```python
from build123d import *

# Parameters (mm, degrees)
SKETCH_1_R           = 11
EXTRUDE_1_DEPTH      = 50
SKETCH_2_R           = 7.5
CUT_EXTRUDE_1_DEPTH  = 53.364109846
SKETCH_4_R           = 1.935
CUT_EXTRUDE_4_DEPTH  = 50
EXTRUDE_3_DEPTH      = 10
EXTRUDE_3_DEPTH_BACK = 3
SKETCH_11_W          = 22
SKETCH_11_H          = 22.065


with BuildPart() as part:
    # 草圖1 → 填料-伸長1 (new body)
    with BuildSketch(Plane(origin=(0, 0, 0), x_dir=(1, 0, 0), z_dir=(0, 1, 0))):
        with Locations(Location((0, 0, 0), (0, 0, 270))):
            Circle(SKETCH_1_R)
    extrude(amount=EXTRUDE_1_DEPTH)

    # 草圖2 → 除料-伸長1 (cut, through all)
    with BuildSketch(Plane(origin=(0, 50, 0), x_dir=(1, 0, 0), z_dir=(0, 1, 0))):
        with Locations(Location((0, 0, 0), (0, 0, 270))):
            Circle(SKETCH_2_R)
    extrude(amount=-CUT_EXTRUDE_1_DEPTH, mode=Mode.SUBTRACT)

    # 草圖4 → 除料-伸長4 (cut)
    with BuildSketch(Plane.XY.offset(12)):
        with Locations((0, 40)):
            Circle(SKETCH_4_R)
    extrude(amount=-CUT_EXTRUDE_4_DEPTH, mode=Mode.SUBTRACT)

    # 草圖11 → 填料-伸長3 (add, two sides: drawn at the far end of the back side and taken through both)
    with BuildSketch(Plane.XY.offset(12).offset(-EXTRUDE_3_DEPTH_BACK)):
        with Locations((0, 11.0325)):
            Rectangle(SKETCH_11_W, SKETCH_11_H)
    extrude(amount=EXTRUDE_3_DEPTH + EXTRUDE_3_DEPTH_BACK)


solid = part.part
```
Input: part model. Units: mm. Frame: model coordinates. Round coordinates to 2 decimals unless told otherwise and drop trailing zeros. Write each loop counter-clockwise with the first axis right and the second up, starting at its lowest first coordinate (ties: lowest second). Pieces come first, ordered by that corner, then holes. Notation, with made-up numbers: (49, -34) -> (65, -34) arc R26 ccw to (65, -10) -> close; hole circle Ø6 at (54, -29). An arc over 180 degrees is marked (long way). Answer as CSV lines item,"result".
1. Mould query, pull axis Z, two halves, no side actions, for faces 1 (the flat face through (2.6, 50, 7.2)), 2 (the flat face through (-9, 11, 9)), 3 (the flat face through (0, 11, 22)). Classes: +Z half, -Z half, draft (parallel to the pull), parting line (faces both ways), or undercut.
Geometry says:
face 1,"draft"
face 2,"undercut"
face 3,"+Z half"
2. Contact query for flat-ended pins moving along their axis: P1, Ø10, axis at x = 2, z = 14.5, coming from the -Y side; P2, Ø5, axis at x = -7.5, y = 12, coming from the -Z side; P3, Ø4, axis at y = 44, z = 10.5, coming from the -X side; P4, Ø2.5, axis at x = 9.5, y = 8, coming from the -Z side. Output: stop coordinate, or through.
Geometry says:
P1,"stops at y = 0"
P2,"stops at z = -9.8"
P3,"stops at x = -6.98"
P4,"stops at z = -7.28"
3. Section D-D (y = 40). Return the cut outline in (x, z) (3 decimals), plus the area to 3 significant figures.
Geometry says:
outline,"(-1.935, -10.828) -> (-1.935, -7.246) arc R7.5 cw to (-1.935, 7.246) -> (-1.935, 10.828) arc R11 ccw to start; (1.935, -10.828) arc R11 ccw to (1.935, 10.828) -> (1.935, 7.246) arc R7.5 cw to (1.935, -7.246) -> close"
area,"176 mm^2"
4. Section A-A (x = 0). Return the cut outline in (y, z) (3 decimals).
Geometry says:
outline,"(0, -11) -> (38.065, -11) -> (38.065, -7.5) -> (0, -7.5) -> close; (0, 7.5) -> (38.065, 7.5) -> (38.065, 11) -> (22.065, 11) -> (22.065, 22) -> (0, 22) -> close; (41.935, -11) -> (50, -11) -> (50, -7.5) -> (41.935, -7.5) -> close; (41.935, 7.5) -> (50, 7.5) -> (50, 11) -> (41.935, 11) -> close"
5. Ray query, L1, parallel to Y at x = 0, z = 9.75 (3 decimals); L2, parallel to Y at x = -1, z = 14 (3 decimals); L3, parallel to X at y = 4, z = 3. Return the intervals inside material, ascending. Write a range as [from, to].
Geometry says:
L1,"y = [0, 38.065], [41.935, 50]"
L2,"y = [0, 22.065]"
L3,"x = [-10.58, -6.87], [6.87, 10.58]"
6. Section C-C (y = 19). Return the cut outline in (x, z).
Geometry says:
outline,"(-11, 9) -> (-6.32, 9) arc R11 ccw (long way) to (6.32, 9) -> (11, 9) -> (11, 22) -> (-11, 22) -> close; hole circle Ø15 at (0, 0)"
7. Section B-B (z = 0). Return the cut outline in (x, y), plus the area to 3 significant figures.
Geometry says:
outline,"(-11, 0) -> (-7.5, 0) -> (-7.5, 50) -> (-11, 50) -> close; (7.5, 0) -> (11, 0) -> (11, 50) -> (7.5, 50) -> close"
area,"350 mm^2"
